from build123d import *

# Parameters (mm, degrees)
EXTRUDE_1_DEPTH          = 34.55
SKETCH_2_W               = 40
SKETCH_2_H               = 8
CUT_EXTRUDE_1_DEPTH      = 16
CHAMFER_1_SIZE           = 2
SKETCH_6_R               = 1.6
EXTRUDE_2_DEPTH          = 6.9
SKETCH_8_R               = 1.6
EXTRUDE_3_DEPTH          = 5.5
CUT_EXTRUDE_6_DEPTH      = 10
CUT_EXTRUDE_7_DEPTH      = 25
CUT_EXTRUDE_8_DEPTH      = 25
CUT_EXTRUDE_8_DEPTH_BACK = 25
SKETCH_14_W              = 20
SKETCH_14_H              = 10
CUT_EXTRUDE_9_DEPTH      = 25
FILLET_1_R               = 2
EXTRUDE_START            = -6
EXTRUDE_4_DEPTH          = 22.55
FILLET_2_R               = 1


with BuildPart() as part:
    # 草图1 → 凸台-拉伸1 (new body)
    with BuildSketch(Plane.XY):
        Polygon((0, 0), (22.5, 0), (22.5, 12), (-22.5, 12), (-22.5, 0), align=None)
    extrude(amount=EXTRUDE_1_DEPTH)

    # 草图2 → 切除-拉伸1 (cut)
    with BuildSketch(Plane.XY.offset(34.55)):
        with Locations((0, 8)):
            Rectangle(SKETCH_2_W, SKETCH_2_H)
    extrude(amount=-CUT_EXTRUDE_1_DEPTH, mode=Mode.SUBTRACT)

    # 倒角1
    chamfer_1_edges = [part.edges().sort_by_distance(p)[0] for p in [
        (20, 4, 26.55),
        (-20, 4, 26.55),
    ]]
    chamfer(chamfer_1_edges, length=CHAMFER_1_SIZE)

    # 草图6 → 凸台-拉伸2 (add)
    with BuildSketch(Plane(origin=(0, 12, 0), x_dir=(1, 0, 0), z_dir=(0, 1, 0))):
        with BuildLine():
            Line((22.5, 0), (22.5, -13.5))
            Line((22.5, -13.5), (17, -13.5))
            ThreePointArc((17, -13.5), (15.232233047, -12.767766953), (14.5, -11))
            Line((14.5, -11), (14.5, -5))
            Line((14.5, -5), (14.5, 0))
            Line((14.5, 0), (22.5, 0))
        make_face()
        with Locations((17, -5)):
            Circle(SKETCH_6_R, mode=Mode.SUBTRACT)
        with Locations((17, -11)):
            Circle(SKETCH_6_R, mode=Mode.SUBTRACT)
        with BuildLine():
            Line((-14.5, 0), (-22.5, 0))
            Line((-22.5, 0), (-22.5, -13.5))
            Line((-22.5, -13.5), (-17, -13.5))
            ThreePointArc((-17, -13.5), (-15.232233047, -12.767766953), (-14.5, -11))
            Line((-14.5, -11), (-14.5, -5))
            Line((-14.5, -5), (-14.5, 0))
        make_face()
        with Locations((-17, -11)):
            Circle(SKETCH_6_R, mode=Mode.SUBTRACT)
        with Locations((-17, -5)):
            Circle(SKETCH_6_R, mode=Mode.SUBTRACT)
    extrude(amount=-EXTRUDE_2_DEPTH)

    # 草图8 → 凸台-拉伸3 (add)
    with BuildSketch(Plane.XY.offset(34.55)):
        with BuildLine():
            Line((1.843049286, -25.367101461), (9.230566594, -19.615105309))
            ThreePointArc((9.230566594, -19.615105309), (9.814108465, -18.625953935), (10.421644381, -17.651355727))
            Line((10.421644381, -17.651355727), (5.476763257, -11.300448334))
            ThreePointArc((5.476763257, -11.300448334), (6.699551666, -1.476763257), (16.523236743, -2.699551666))
            Line((16.523236743, -2.699551666), (19.967990067, -6.846461039))
            ThreePointArc((19.967990067, -6.846461039), (22.224318463, -5.085470923), (24.58365332, -3.465087309))
            ThreePointArc((24.58365332, -3.465087309), (26.278709649, -3.148232211), (27.365383934, -1.809295278))
            ThreePointArc((27.365383934, -1.809295278), (28.658809968, -1.124546474), (29.972928279, -0.480399834))
            ThreePointArc((29.972928279, -0.480399834), (29.349734714, 1.46572665), (28, 3))
            Line((28, 3), (22.5, 3))
            Line((22.5, 3), (22.5, 4))
            Line((22.5, 4), (-22.5, 4))
            Line((-22.5, 4), (-22.5, 3))
            Line((-22.5, 3), (-28, 3))
            ThreePointArc((-28, 3), (-29.349734714, 1.46572665), (-29.972928279, -0.480399834))
            ThreePointArc((-29.972928279, -0.480399834), (-28.658809968, -1.124546474), (-27.365383934, -1.809295278))
            ThreePointArc((-27.365383934, -1.809295278), (-26.278709649, -3.148232211), (-24.58365332, -3.465087309))
            ThreePointArc((-24.58365332, -3.465087309), (-22.224318463, -5.085470923), (-19.967990067, -6.846461039))
            Line((-19.967990067, -6.846461039), (-16.523236743, -2.699551666))
            ThreePointArc((-16.523236743, -2.699551666), (-6.699551666, -1.476763257), (-5.476763257, -11.300448334))
            Line((-5.476763257, -11.300448334), (-10.421644381, -17.651355727))
            ThreePointArc((-10.421644381, -17.651355727), (-9.814108465, -18.625953935), (-9.230566594, -19.615105309))
            Line((-9.230566594, -19.615105309), (-1.843049286, -25.367101461))
            ThreePointArc((-1.843049286, -25.367101461), (0, -26), (1.843049286, -25.367101461))
        make_face()
        with Locations((25, -1)):
            Circle(SKETCH_8_R, mode=Mode.SUBTRACT)
        with Locations((0, -23)):
            Circle(SKETCH_8_R, mode=Mode.SUBTRACT)
        with Locations((-25, -1)):
            Circle(SKETCH_8_R, mode=Mode.SUBTRACT)
    extrude(amount=-EXTRUDE_3_DEPTH)

    # 草图11 → 切除-拉伸6 (cut)
    with BuildSketch(Plane(origin=(0, 0, 29.05), x_dir=(-1, 0, 0), z_dir=(0, 0, -1))):
        Polygon((-4, -7), (-10.421644381, -17.651355727), (-10.421644381, -27.0891889), (10.421644381, -27.0891889), (10.421644381, -17.651355727), (4, -7), (5.255437353, -3), (0, -3), (-5.255437353, -3), align=None)
    extrude(amount=-CUT_EXTRUDE_6_DEPTH, mode=Mode.SUBTRACT)

    # 草图12 → 切除-拉伸7 (cut)
    with BuildSketch(Plane.XY.offset(18.55)):
        Polygon((-18, 6), (-16, 4), (16, 4), (18, 6), (18, 12), (-18, 12), align=None)
    extrude(amount=-CUT_EXTRUDE_7_DEPTH, mode=Mode.SUBTRACT)

    # 草图13 → 切除-拉伸8 (cut, two sides)
    with BuildSketch(Plane(origin=(0, 4, 0), x_dir=(1, 0, 0), z_dir=(0, 1, 0))) as cut_extrude_8_sk:
        Polygon((-7.75, -24.45), (-7.75, -28.45), (-7.75, -29.45), (-22.5, -29.45), (-22.5, -28.45), (-22.5, -24.45), (-22.5, -21.45), (-22.5, -19.45), (-7.75, -19.45), align=None)
        Polygon((22.5, -19.45), (22.5, -21.45), (22.5, -24.45), (22.5, -28.45), (22.5, -29.45), (7.75, -29.45), (7.75, -28.45), (7.75, -24.45), (7.75, -19.45), align=None)
    extrude(amount=CUT_EXTRUDE_8_DEPTH, mode=Mode.SUBTRACT)
    extrude(cut_extrude_8_sk.sketch, amount=-CUT_EXTRUDE_8_DEPTH_BACK, mode=Mode.SUBTRACT)

    # 草图14 → 切除-拉伸9 (cut)
    with BuildSketch(Plane(origin=(0, 4, 0), x_dir=(1, 0, 0), z_dir=(0, 1, 0))):
        with Locations((0, -5)):
            Rectangle(SKETCH_14_W, SKETCH_14_H)
    extrude(amount=-CUT_EXTRUDE_9_DEPTH, mode=Mode.SUBTRACT)

    # 圆角1
    fillet_1_edges = [part.edges().sort_by_distance(p)[0] for p in [
        (10, 2, 0),
        (-10, 2, 0),
        (10, 2, 10),
        (-10, 2, 10),
    ]]
    fillet(fillet_1_edges, radius=FILLET_1_R)

    # 草图15 → 凸台-拉伸4 (add)
    with BuildSketch(Plane(origin=(0, 0, 0), x_dir=(-1, 0, 0), z_dir=(0, 0, -1)).offset(EXTRUDE_START)):
        with BuildLine():
            Line((-22.5, 9.5), (-22.5, 3))
            Line((-22.5, 3), (-32.5, 3))
            Line((-32.5, 3), (-32.5, -0.458843457))
            ThreePointArc((-32.5, -0.458843457), (-42.310755549, 2.352789548), (-52.5, 2.932014979))
            Line((-52.5, 2.932014979), (-52.5, 9.5))
            Line((-52.5, 9.5), (-22.5, 9.5))
        make_face()
        with BuildLine():
            Line((-24.5, 7.5), (-24.5, 5))
            Line((-24.5, 5), (-34.5, 5))
            Line((-34.5, 5), (-34.5, 2.428515274))
            ThreePointArc((-34.5, 2.428515274), (-42.390809061, 4.393039713), (-50.5, 4.997395763))
            Line((-50.5, 4.997395763), (-50.5, 7.5))
            Line((-50.5, 7.5), (-24.5, 7.5))
        make_face(mode=Mode.SUBTRACT)
        with BuildLine():
            Line((32.5, 3), (32.5, -0.458843457))
            ThreePointArc((32.5, -0.458843457), (42.310755549, 2.352789548), (52.5, 2.932014979))
            Line((52.5, 2.932014979), (52.5, 9.5))
            Line((52.5, 9.5), (22.5, 9.5))
            Line((22.5, 9.5), (22.5, 3))
            Line((22.5, 3), (32.5, 3))
        make_face()
        with BuildLine():
            Line((24.5, 7.5), (50.5, 7.5))
            Line((50.5, 7.5), (50.5, 4.997395763))
            ThreePointArc((50.5, 4.997395763), (42.390809061, 4.393039713), (34.5, 2.428515274))
            Line((34.5, 2.428515274), (34.5, 5))
            Line((34.5, 5), (24.5, 5))
            Line((24.5, 5), (24.5, 7.5))
        make_face(mode=Mode.SUBTRACT)
    extrude(amount=-EXTRUDE_4_DEPTH)

    # 圆角2
    fillet_2_edges = [part.edges().sort_by_distance(p)[0] for p in [
        (52.5, 9.5, 17.275),
        (32.5, 3, 17.275),
        (32.5, -0.458843457, 17.275),
        (52.5, 2.932014979, 17.275),
        (24.5, 7.5, 17.275),
        (24.5, 5, 17.275),
        (34.5, 5, 17.275),
        (34.5, 2.428515274, 17.275),
        (50.5, 4.997395763, 17.275),
        (50.5, 7.5, 17.275),
        (-52.5, 9.5, 17.275),
        (-52.5, 2.932014979, 17.275),
        (-32.5, -0.458843457, 17.275),
        (-32.5, 3, 17.275),
        (-24.5, 7.5, 17.275),
        (-50.5, 7.5, 17.275),
        (-50.5, 4.997395763, 17.275),
        (-34.5, 2.428515274, 17.275),
        (-34.5, 5, 17.275),
        (-24.5, 5, 17.275),
    ]]
    fillet(fillet_2_edges, radius=FILLET_2_R)


solid = part.part
Work out the finished part from the listing and answer in its coordinate system (mm). A direction names the side the tool comes from. Round coordinates to 2 decimals unless told otherwise and drop trailing zeros. Order: outer loops, then holes, each group sorted by start corner. A loop starts at its lowest first (then second) coordinate and runs counter-clockwise, first axis right, second up. Notation, with made-up numbers: M 7.25,25.5 L 63.25,25.5 A20 cw 63.25,60.5 Z; hole C -12.75,20.25 d3. An arc over 180 degrees is marked long. Put each result on its own line as item: value. Start each with the question number.
Q1. For a pull along Y with two mould halves and no side action, classify faces 5 (the flat face through (17, 5, 9)), 6 (the flat face through (-10, 2, 5)), 7 (the flat face through (-30, 5, 17)), 8 (the cylindrical face through (11, 0, 32)) as pulls with the +Y half, pulls with the -Y half, needs draft (parallel to the pull), parting line crosses it, or undercut.
Q2. Flat-ended cylindrical pins translate along their axes: pin 1 (8 mm diameter, centred on x = -41.5, z = 8, fed in from +Y); pin 2 (6 mm diameter, centred on x = 29, y = -1, fed in from -Z); pin 3 (1 mm diameter, centred on x = 9.5, z = 13, fed in from -Y). Find the tip coordinate at first contact, or state that the pin passes through.
Q3. Section C-C, the plane z = 5 is taken. Write down the section's boundary in (x, y), and give its area (3 significant figures).
Q4. Section D-D, the plane x = -2 is taken. Write down the section's boundary in (y, z), and give its area (3 significant figures).
Q5. Section B-B, the plane x = 13 is taken. Write down the section's boundary in (y, z).
Q6. Section A-A, the plane z = 31.5 is taken. Write down the section's boundary in (x, y), and give its area (3 significant figures).
Q7. Straight lines are drawn through the part: L1, parallel to Y at x = -25, z = 31.8; L2, parallel to X at y = 7.5, z = 2.5; L3, parallel to X at y = 3.25, z = 2. For each, find the intervals that lie inside material, in ascending order. Write a range as [from, to].
Q8. A tool of negligible diameter and unlimited length cuts with its end or side. For faces 1 (the flat face through (-37, 8, 28.55)), 2 (the flat face through (-17, 3, 19.45)), 3 (the cylindrical face through (-10.57, 1.97, 0.6)), 4 (the flat face through (19, 5, 32)), from which of +Z, -Z, +X, -X, +Y, -Y can it reach the whole face along a straight path? Write none if from no direction.
Findings below:
1. face 5: pulls with the +Y half
1. face 6: needs draft
1. face 7: undercut
1. face 8: pulls with the -Y half
2. pin 1: stops at y = 9.5
2. pin 2: stops at z = 29.05
2. pin 3: stops at y = 0
3. outline: M -22.5,0 L -10,0 L -10,4 L -16,4 L -18,6 L -18,12 L -22.5,12 Z; M 10,0 L 22.5,0 L 22.5,12 L 18,12 L 18,6 L 16,4 L 10,4 Z
3. area: 176 mm^2
4. outline: M -3,29.05 L 0,29.05 L 0,10 L 4,10 L 4,34.55 L -3,34.55 Z
4. area: 115 mm^2
5. outline: M -0.29,29.45 L 4,29.45 L 4,34.55 L -0.29,34.55 Z; M 0,0 L 4,0 L 4,19.45 L 0,19.45 Z
6. outline: M -29.97,-0.48 A47 cw -27.37,-1.81 A2.5 ccw -24.58,-3.47 A47 cw -19.97,-6.85 L -16.52,-2.7 A7 cw -5.26,-3 L 5.26,-3 A7 cw 16.52,-2.7 L 19.97,-6.85 A47 cw 24.58,-3.47 A2.5 ccw 27.37,-1.81 A47 cw 29.97,-0.48 A5 ccw 28,3 L 22.5,3 L 22.5,12 L 20,12 L 20,6 L 18,4 L -18,4 L -20,6 L -20,12 L -22.5,12 L -22.5,3 L -28,3 A5 ccw Z; hole C -25,-1 d3.2; hole C 25,-1 d3.2
6. area: 402 mm^2
7. L1: y = [-3.5, -2.6], [0.6, 3]
7. L2: x = [-22.5, -18], [18, 22.5]
7. L3: x = [-22.5, -10], [10, 22.5]
8. face 1: +Z, -X, +Y, -Y
8. face 2: +Y, -Y
8. face 3: -Z, +Y, -Y
8. face 4: +Z, +Y
